from build123d import *

# Parameters (mm, degrees)
BOSS_EXTRUDE1_DEPTH = 4.5


with BuildPart() as part:
    # Sketch1 → Boss-Extrude1 (new body)
    with BuildSketch(Plane(origin=(0, 0, 0), x_dir=(1, 0, 0), z_dir=(0, 1, 0))):
        with BuildLine():
            Line((-6, 0), (-6, -5))
            Line((-6, -5), (-6, -16.5))
            ThreePointArc((-6, -16.5), (-5.414213562, -17.914213562), (-4, -18.5))
            Line((-4, -18.5), (4, -18.5))
            ThreePointArc((4, -18.5), (5.414213562, -17.914213562), (6, -16.5))
            Line((6, -16.5), (6, -5))
            Line((6, -5), (6, 0))
            ThreePointArc((6, 0), (0, 6), (-6, 0))
        make_face()
        with BuildLine():
            Line((3, 0), (3, -2))
            ThreePointArc((3, -2), (2.904829219, -2.773082305), (2.625, -3.5))
            ThreePointArc((2.625, -3.5), (2.345170781, -4.226917695), (2.25, -5))
            Line((2.25, -5), (2.25, -13.133974596))
            ThreePointArc((2.25, -13.133974596), (2.316987298, -13.383974596), (2.5, -13.566987298))
            ThreePointArc((2.5, -13.566987298), (2.732962913, -14.129409523), (2.25, -14.5))
            Line((2.25, -14.5), (-2.25, -14.5))
            ThreePointArc((-2.25, -14.5), (-2.732962913, -14.129409523), (-2.5, -13.566987298))
            ThreePointArc((-2.5, -13.566987298), (-2.316987298, -13.383974596), (-2.25, -13.133974596))
            Line((-2.25, -13.133974596), (-2.25, -5))
            ThreePointArc((-2.25, -5), (-2.345170781, -4.226917695), (-2.625, -3.5))
            ThreePointArc((-2.625, -3.5), (-2.904829219, -2.773082305), (-3, -2))
            Line((-3, -2), (-3, 0))
            ThreePointArc((-3, 0), (0, 3), (3, 0))
        make_face(mode=Mode.SUBTRACT)
    extrude(amount=BOSS_EXTRUDE1_DEPTH)


solid = part.part
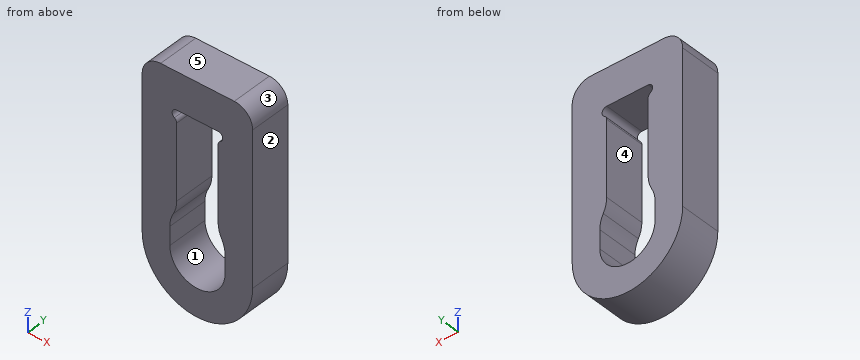
Here's how the part is built. I have some questions about the finished solid (model axes, mm). Face numbers are marked on the shaded views. A direction names the side the tool comes from. Round coordinates to 2 decimals unless told otherwise and drop trailing zeros. Order: outer loops, then holes, each group sorted by start corner. A loop starts at its lowest first (then second) coordinate and runs counter-clockwise, first axis right, second up. Notation, with made-up numbers: M 25,3 L 48,3 A21 cw 48,18 Z; hole C 83.25,36.25 d5. An arc over 180 degrees is marked long. One line per question, with ' | ' between items.
1) On a 3-axis mill with a long thin cutter (end or side, diameter ignored), from which of +Z, -Z, +X, -X, +Y, -Y can I reach the whole of each face in a straight line? I mean the marked faces 1 and 2. Say none if no direction works.
Checked values:
face 1: +Y, -Y | face 2: +Z, -Z, +X, +Y, -Y
2) Imagine slicing it at B-B, the plane z = 11. Write out the boundary of the cut face in (x, y).
Checked values:
outline: M -6,0 L -2.25,0 L -2.25,4.5 L -6,4.5 Z; M 2.25,0 L 6,0 L 6,4.5 L 2.25,4.5 Z
3) I need wall thicknesses on line 1 (X direction, y = 1, z = 10.5); line 2 (X direction, y = 3.2, z = 1.75); line 3 (Z direction, x = -1, y = 4). Which ranges of each line are inside material? Lowest first, please.
Checked values:
line 1: x = -6 to -2.25, 2.25 to 6 | line 2: x = -6 to -3, 3 to 6 | line 3: z = -5.92 to -2.83, 14.5 to 18.5
4) We'd pull the mould along X, two halves only. Please class the marked faces 3, 4 and 5: released by +X, released by -X, zero draft, split by the parting line, or undercut.
Checked values:
face 3: released by +X | face 4: undercut | face 5: zero draft
5) I'm going to push a flat-ended pin straight in: pin 1 Ø1 at (y, z) = (2, -2) entering from -X. Where does the tip first touch, or does it pass through?
Checked values:
pin 1: stops at x = -5.81
6) Imagine slicing it at A-A, the plane x = 0. Write out the boundary of the cut face in (y, z), plus the area to 3 significant figures.
Checked values:
outline: M 0,-6 L 4.5,-6 L 4.5,-3 L 0,-3 Z; M 0,14.5 L 4.5,14.5 L 4.5,18.5 L 0,18.5 Z | area: 31.5 mm²
7) Imagine slicing it at D-D, the plane x = -4.25. Write out the boundary of the cut face in (y, z).
Checked values:
outline: M 0,-4.24 L 4.5,-4.24 L 4.5,18.48 L 0,18.48 Z
